Input: part model. Units: mm. Frame: model coordinates. A direction names the side the tool comes from. Round coordinates to 2 decimals unless told otherwise and drop trailing zeros. Order: outer loops, then holes, each group sorted by start corner. A loop starts at its lowest first (then second) coordinate and runs counter-clockwise, first axis right, second up. Notation, with made-up numbers: (50.25, 17.5) -> (57.25, 17.5) arc R25 ccw to (57.25, 30.5) -> close; hole circle Ø5 at (77, 18). An arc over 180 degrees is marked (long way). Use a Markdown table: item, result.
from build123d import *

# Parameters (mm, degrees)
PAD_DEPTH       = 3
SKETCH001_W     = 26
SKETCH001_H     = 18
PAD001_DEPTH    = 22
SKETCH002_W     = 23
SKETCH002_H     = 15
POCKET_DEPTH    = 23.5
SKETCH003_W     = 20
SKETCH003_H     = 12
POCKET001_DEPTH = 1.501
SKETCH004_R     = 3.5
POCKET002_DEPTH = 25.001
POCKET003_DEPTH = 1.5


with BuildPart() as part:
    # Sketch → Pad (new body)
    with BuildSketch(Plane.XY):
        with BuildLine():
            Line((0, 0), (26, 0))
            Line((26, 0), (26, 18))
            Line((26, 18), (0, 18))
            Line((0, 18), (-8.937931, 16.944828))
            ThreePointArc((-8.937931, 16.944828), (-16, 9), (-8.937931, 1.055172))
            Line((-8.937931, 1.055172), (0, 0))
        make_face()
    extrude(amount=PAD_DEPTH)

    # Sketch001 (on Face8 of Pad) → Pad001 (join)
    with BuildSketch(Plane.XY.offset(3)):
        with Locations((13, 9)):
            Rectangle(SKETCH001_W, SKETCH001_H)
    extrude(amount=PAD001_DEPTH)

    # Sketch002 (on Face2 of Pad001) → Pocket (cut)
    with BuildSketch(Plane(origin=(0, 0, 0), x_dir=(1, 0, 0), z_dir=(0, 0, -1))):
        with Locations((13, -9)):
            Rectangle(SKETCH002_W, SKETCH002_H)
    extrude(amount=-POCKET_DEPTH, mode=Mode.SUBTRACT)

    # Sketch003 (on Face15 of Pocket) → Pocket001 (cut, through all)
    with BuildSketch(Plane(origin=(0, 0, 23.5), x_dir=(1, 0, 0), z_dir=(0, 0, -1))):
        with Locations((13, -9)):
            Rectangle(SKETCH003_W, SKETCH003_H)
    extrude(amount=-POCKET001_DEPTH, mode=Mode.SUBTRACT)

    # Sketch004 (on Face4 of Pocket001) → Pocket002 (cut, through all)
    with BuildSketch(Plane(origin=(0, 0, 0), x_dir=(1, 0, 0), z_dir=(0, 0, -1))):
        with Locations((-8, -9)):
            Circle(SKETCH004_R)
    extrude(amount=-POCKET002_DEPTH, mode=Mode.SUBTRACT)

    # Sketch005 (on Face7 of Pocket002) → Pocket003 (cut)
    with BuildSketch(Plane.YZ.offset(26)):
        Polygon((12.5, 0), (9, 6.062178), (5.5, 0), align=None)
    extrude(amount=-POCKET003_DEPTH, mode=Mode.SUBTRACT)


solid = part.part
1) Pin query (flat end, axial travel): pin 1 Ø8 at (y, z) = (11.5, 16.5) entering from -X; pin 2 Ø5 at (x, y) = (14.5, 6.5) entering from -Z; pin 3 Ø5 at (x, y) = (-10, 11) entering from +Z; pin 4 Ø12 at (x, z) = (2.5, 5.5) entering from -Y. Return the tip coordinate at first contact, or that it passes through.
Results found:
| item | result |
|---|---|
| pin 1 | stops at x = 0 |
| pin 2 | passes through |
| pin 3 | stops at z = 3 |
| pin 4 | stops at y = 0 |
2) Pull-direction query (X, two-part tool) for faces 5 (the flat face through (0, 9, 14)), 6 (the flat face through (26, 9, 12)), 7 (the flat face through (13, 1.5, 12)); classes: +X half, -X half, draft (parallel to the pull), parting line (faces both ways), or undercut.
Results found:
| item | result |
|---|---|
| face 5 | -X half |
| face 6 | +X half |
| face 7 | undercut |
3) Cut plane D-D on y = 4.5. Return loops of the section in (x, z), and give its area (3 significant figures).
Results found:
| item | result |
|---|---|
| outline | (-14.61, 0) -> (1.5, 0) -> (1.5, 23.5) -> (3, 23.5) -> (3, 25) -> (0, 25) -> (0, 3) -> (-14.61, 3) -> close; (23, 23.5) -> (24.5, 23.5) -> (24.5, 0) -> (26, 0) -> (26, 25) -> (23, 25) -> close |
| area | 123 mm² |
4) Cut plane B-B on y = 6.5. Return loops of the section in (x, z), and give its area (3 significant figures).
Results found:
| item | result |
|---|---|
| outline | (-15.6, 0) -> (-10.45, 0) -> (-10.45, 3) -> (-15.6, 3) -> close; (-5.55, 0) -> (1.5, 0) -> (1.5, 23.5) -> (3, 23.5) -> (3, 25) -> (0, 25) -> (0, 3) -> (-5.55, 3) -> close; (23, 23.5) -> (24.5, 23.5) -> (24.5, 1.73) -> (26, 1.73) -> (26, 25) -> (23, 25) -> close |
| area | 109 mm² |
5) Line query: L1, parallel to X at y = 4.25, z = 9; L2, parallel to Y at x = 22, z = 1.25; L3, parallel to X at y = 9, z = 2.35. Output: solid intervals per line, ascending. Write a range as [from, to].
Results found:
| item | result |
|---|---|
| L1 | x = [0, 1.5], [24.5, 26] |
| L2 | y = [0, 1.5], [16.5, 18] |
| L3 | x = [-16, -11.5], [-4.5, 1.5] |
6) Cut plane C-C on z = 19. Return loops of the section in (x, y).
Results found:
| item | result |
|---|---|
| outline | (0, 0) -> (26, 0) -> (26, 18) -> (0, 18) -> close; hole (1.5, 1.5) -> (24.5, 1.5) -> (24.5, 16.5) -> (1.5, 16.5) -> close |
7) Cut plane A-A on x = 5.5. Return loops of the section in (y, z), and give its area (3 significant figures).
Results found:
| item | result |
|---|---|
| outline | (0, 0) -> (1.5, 0) -> (1.5, 23.5) -> (3, 23.5) -> (3, 25) -> (0, 25) -> close; (15, 23.5) -> (16.5, 23.5) -> (16.5, 0) -> (18, 0) -> (18, 25) -> (15, 25) -> close |
| area | 79.5 mm² |
8) Set-up query: faces 1 (the flat face through (25.26, 7.274, 3.074)), 2 (the flat face through (13, 2, 23.5)), 3 (the flat face through (13, 15, 24)), 4 (the flat face through (-4.6, 7.1, 3)). Return all of +Z, -Z, +X, -X, +Y, -Y with unobstructed straight access to the full face (end or side cutting, diameter ignored); none if empty.
Results found:
| item | result |
|---|---|
| face 1 | -Z, +X |
| face 2 | -Z |
| face 3 | +Z, -Z |
| face 4 | +Z, -X, +Y, -Y |
